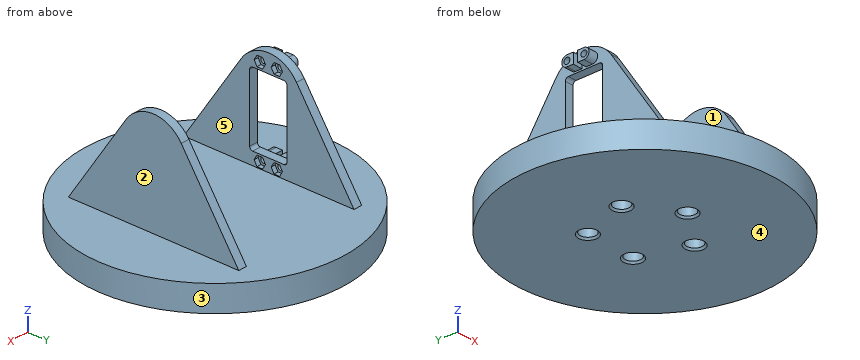
```python
from build123d import *

# Parameters (mm, degrees)
SKETCH1_R           = 75
BASE_PLATE_DEPTH    = 15
SKETCH2_R           = 4.5
DRIVE_HOLES_DEPTH   = 10
CHAMFER1_SIZE       = 1
BASE_START          = 40
BASE_FIN_DEPTH      = 5
BASE_START_2        = 70
BASE_FIN_2_DEPTH    = 5
CUT_EXTRUDE1_REACH  = 158.203
CUT_EXTRUDE2_REACH  = 158.203
SKETCH7_R           = 1.75
BOSS_EXTRUDE1_DEPTH = 5.6
CUT_EXTRUDE3_START  = -5.6
SKETCH9_R           = 1.75
CUT_EXTRUDE3_DEPTH  = 5.6
SKETCH10_W          = 4.6
SKETCH10_H          = 2.5
SKETCH10_W_2        = 6
CUT_EXTRUDE4_DEPTH  = 5.6
CUT_EXTRUDE5_DEPTH  = 2.6


with BuildPart() as part:
    # Sketch1 → Base Plate (new body)
    with BuildSketch(Plane.XY):
        Circle(SKETCH1_R)
    extrude(amount=BASE_PLATE_DEPTH)

    # Sketch2 → Drive Holes (cut)
    with BuildSketch(Plane(origin=(0, 0, 0), x_dir=(-1, 0, 0), z_dir=(0, 0, -1))):
        with Locations((0, -25)):
            Circle(SKETCH2_R)
        with Locations((-23.776412907, -7.725424859)):
            Circle(SKETCH2_R)
        with Locations((-14.694631307, 20.225424859)):
            Circle(SKETCH2_R)
        with Locations((14.694631307, 20.225424859)):
            Circle(SKETCH2_R)
        with Locations((23.776412907, -7.725424859)):
            Circle(SKETCH2_R)
    extrude(amount=-DRIVE_HOLES_DEPTH, mode=Mode.SUBTRACT)

    # Chamfer1
    chamfer1_edges = [part.edges().sort_by_distance(p)[0] for p in [
        (28.276412907, -7.725424859, 0),
        (19.194631307, 20.225424859, 0),
        (-10.194631307, 20.225424859, 0),
        (-19.276412907, -7.725424859, 0),
        (4.5, -25, 0),
    ]]
    chamfer(chamfer1_edges, length=CHAMFER1_SIZE)

    # Sketch4 → Base Fin (add)
    with BuildSketch(Plane(origin=(0, 0, 0), x_dir=(0, 0, -1), z_dir=(1, 0, 0)).offset(BASE_START)):
        with BuildLine():
            Line((-15, 50), (-65.791986374, 16.233382914))
            ThreePointArc((-65.791986374, 16.233382914), (-74.493324261, 0), (-65.791986374, -16.233382914))
            Line((-65.791986374, -16.233382914), (-15, -50))
            Line((-15, -50), (-15, 50))
        make_face()
    extrude(amount=-BASE_FIN_DEPTH)

    # Sketch5 → Base Fin 2 (add)
    with BuildSketch(Plane.ZY.offset(-35).offset(BASE_START_2)):
        with BuildLine():
            Line((15, 50), (15, -50))
            Line((15, -50), (65.791986374, -16.233382914))
            ThreePointArc((65.791986374, -16.233382914), (74.493324261, 0), (65.791986374, 16.233382914))
            Line((65.791986374, 16.233382914), (15, 50))
        make_face()
    extrude(amount=BASE_FIN_2_DEPTH)

    # Sketch6 → Cut-Extrude1 (cut, up to next)
    with BuildSketch(Plane.ZY.offset(40), mode=Mode.PRIVATE) as cut_extrude1_sk1:
        with BuildLine():
            Line((64, 8.875345998), (64, -9.524654002))
            ThreePointArc((64, -9.524654002), (63.487436867, -10.762090869), (62.25, -11.274654002))
            Line((62.25, -11.274654002), (24.05, -11.274654002))
            ThreePointArc((24.05, -11.274654002), (22.812563133, -10.762090869), (22.3, -9.524654002))
            Line((22.3, -9.524654002), (22.3, 8.875345998))
            ThreePointArc((22.3, 8.875345998), (22.812563133, 10.112782865), (24.05, 10.625345998))
            Line((24.05, 10.625345998), (62.25, 10.625345998))
            ThreePointArc((62.25, 10.625345998), (63.487436867, 10.112782865), (64, 8.875345998))
        make_face()
    cut_extrude1_tool1 = extrude(cut_extrude1_sk1.sketch, amount=-CUT_EXTRUDE1_REACH, mode=Mode.PRIVATE) & part.part
    add(cut_extrude1_tool1.solids().sort_by_distance((-40, -0.324654, 43.15))[0], mode=Mode.SUBTRACT)

    # Sketch7 → Cut-Extrude2 (cut, up to next)
    with BuildSketch(Plane.ZY.offset(40), mode=Mode.PRIVATE) as cut_extrude2_sk1:
        with Locations((18.35, 4.675345998)):
            Circle(SKETCH7_R)
    cut_extrude2_tool1 = extrude(cut_extrude2_sk1.sketch, amount=-CUT_EXTRUDE2_REACH, mode=Mode.PRIVATE) & part.part
    # Sketch7 → Cut-Extrude2 (cut, up to next)
    with BuildSketch(Plane.ZY.offset(40), mode=Mode.PRIVATE) as cut_extrude2_sk2:
        with Locations((18.35, -5.324654002)):
            Circle(SKETCH7_R)
    cut_extrude2_tool2 = extrude(cut_extrude2_sk2.sketch, amount=-CUT_EXTRUDE2_REACH, mode=Mode.PRIVATE) & part.part
    # Sketch7 → Cut-Extrude2 (cut, up to next)
    with BuildSketch(Plane.ZY.offset(40), mode=Mode.PRIVATE) as cut_extrude2_sk3:
        with Locations((67.95, -5.324654002)):
            Circle(SKETCH7_R)
    cut_extrude2_tool3 = extrude(cut_extrude2_sk3.sketch, amount=-CUT_EXTRUDE2_REACH, mode=Mode.PRIVATE) & part.part
    # Sketch7 → Cut-Extrude2 (cut, up to next)
    with BuildSketch(Plane.ZY.offset(40), mode=Mode.PRIVATE) as cut_extrude2_sk4:
        with Locations((67.95, 4.675345998)):
            Circle(SKETCH7_R)
    cut_extrude2_tool4 = extrude(cut_extrude2_sk4.sketch, amount=-CUT_EXTRUDE2_REACH, mode=Mode.PRIVATE) & part.part
    add(cut_extrude2_tool1.solids().sort_by_distance((-40, 4.675346, 18.35))[0], mode=Mode.SUBTRACT)
    add(cut_extrude2_tool2.solids().sort_by_distance((-40, -5.324654, 18.35))[0], mode=Mode.SUBTRACT)
    add(cut_extrude2_tool3.solids().sort_by_distance((-40, -5.324654, 67.95))[0], mode=Mode.SUBTRACT)
    add(cut_extrude2_tool4.solids().sort_by_distance((-40, 4.675346, 67.95))[0], mode=Mode.SUBTRACT)

    # Sketch8 → Boss-Extrude1 (add)
    with BuildSketch(Plane.ZY.offset(40)):
        with BuildLine():
            Line((70.95, 4.675345998), (70.95, -5.324654002))
            ThreePointArc((70.95, -5.324654002), (67.95, -8.324654002), (64.95, -5.324654002))
            Line((64.95, -5.324654002), (64.95, 4.675345998))
            ThreePointArc((64.95, 4.675345998), (67.95, 7.675345998), (70.95, 4.675345998))
        make_face()
        with BuildLine():
            Line((15, 7.675345998), (15, 0))
            Line((15, 0), (15, -8.324654002))
            Line((15, -8.324654002), (18.35, -8.324654002))
            ThreePointArc((18.35, -8.324654002), (20.471320344, -7.445974346), (21.35, -5.324654002))
            Line((21.35, -5.324654002), (21.35, 4.675345998))
            ThreePointArc((21.35, 4.675345998), (20.471320344, 6.796666341), (18.35, 7.675345998))
            Line((18.35, 7.675345998), (15, 7.675345998))
        make_face()
    extrude(amount=BOSS_EXTRUDE1_DEPTH)

    # Sketch9 → Cut-Extrude3 (cut)
    with BuildSketch(Plane(origin=(-40, 0, 0), x_dir=(0, 0, -1), z_dir=(1, 0, 0)).offset(CUT_EXTRUDE3_START)):
        with Locations(Location((-67.95, -5.324654002, 0), (0, 0, 180))):
            Circle(SKETCH9_R)
        with Locations(Location((-67.95, 4.675345998, 0), (0, 0, 180))):
            Circle(SKETCH9_R)
        with Locations(Location((-18.35, -5.324654002, 0), (0, 0, 180))):
            Circle(SKETCH9_R)
        with Locations(Location((-18.35, 4.675345998, 0), (0, 0, 180))):
            Circle(SKETCH9_R)
    extrude(amount=CUT_EXTRUDE3_DEPTH, mode=Mode.SUBTRACT)

    # Sketch10 → Cut-Extrude4 (cut)
    with BuildSketch(Plane.ZY.offset(45.6)):
        with Locations((19.05, -0.324654002)):
            Rectangle(SKETCH10_W, SKETCH10_H)
        with Locations((67.95, -0.324654002)):
            Rectangle(SKETCH10_W_2, SKETCH10_H)
    extrude(amount=-CUT_EXTRUDE4_DEPTH, mode=Mode.SUBTRACT)

    # Sketch11 → Cut-Extrude5 (cut)
    with BuildSketch(Plane(origin=(-35, 0, 0), x_dir=(0, 0, -1), z_dir=(1, 0, 0))):
        Polygon((-67.94416086, -2.00489509), (-70.822075983, -3.659717702), (-70.827915123, -6.979476615), (-67.95583914, -8.644412915), (-65.077924017, -6.989590302), (-65.072084877, -3.66983139), align=None)
        Polygon((-67.95, 7.995110046), (-70.825, 6.335228022), (-70.825, 3.015463974), (-67.95, 1.35558195), (-65.075, 3.015463974), (-65.075, 6.335228022), align=None)
        Polygon((-18.353543237, -2.004891845), (-21.226769981, -3.667841457), (-21.223226744, -6.987603614), (-18.346456763, -8.644416159), (-15.473230019, -6.981466547), (-15.476773256, -3.66170439), align=None)
        Polygon((-18.355430794, 7.995105604), (-21.22771155, 6.330522595), (-21.222280756, 3.010762989), (-18.344569206, 1.355586392), (-15.47228845, 3.020169401), (-15.477719244, 6.339929006), align=None)
    extrude(amount=-CUT_EXTRUDE5_DEPTH, mode=Mode.SUBTRACT)


solid = part.part
```
Geometry check sheet. Reference: the model listing, model coordinates, mm. Face numbers are marked on the shaded views. A direction names the side the tool comes from. Coordinates: 2 decimals unless noted, no trailing zeros. Order: outer loops, then holes, each group sorted by start corner. A loop starts at its lowest first (then second) coordinate and runs counter-clockwise, first axis right, second up. Notation, with made-up numbers: (83.5, 37) - (92.5, 37) arc R16 cw to (92.5, 53) - close; hole circle Ø7 at (61, -15.5). An arc over 180 degrees is marked (long way). Use one line per item in the form item = value.
1. Draft check along X on the marked faces 3, 4 and 5. Enter one of: pulls with the +X half, pulls with the -X half, needs draft (parallel to the pull), parting line crosses it, or undercut.
Here are the results:
face_3 = parting line crosses it
face_4 = needs draft
face_5 = undercut
2. Section check B-B (z = 6). Record the boundary of the cut face in (x, y).
Here are the results:
outline = circle Ø150 at (0, 0); hole circle Ø9 at (-23.78, -7.73); hole circle Ø9 at (-14.69, 20.23); hole circle Ø9 at (0, -25); hole circle Ø9 at (14.69, 20.23); hole circle Ø9 at (23.78, -7.73)
3. Section check D-D (x = -32.5). Record the boundary of the cut face in (y, z), then the cut area to 3 significant figures.
Here are the results:
outline = (-67.59, 0) - (67.59, 0) - (67.59, 15) - (-67.59, 15) - close
area = 2,030 mm²
4. Scan lines: line 1 (X direction, y = -44, z = 18); line 2 (Y direction, x = -39.4, z = 18.35); line 3 (Y direction, x = -37, z = 65.5). Record each from-to range of solid material in increasing order.
Here are the results:
line_1 = -40 to -35, 35 to 40
line_2 = -47.77 to -7.07, -3.57 to 2.93, 6.43 to 47.77
line_3 = -16.43 to -7.23, -3.42 to 2.77, 6.58 to 16.43
5. Access from +Z, -Z, +X, -X, +Y, -Y to the whole of each face (thin tool, end or side, straight path). Record for the marked faces 1 and 2.
Here are the results:
face_1 = +Z, +Y, -Y
face_2 = +Z, +X, +Y, -Y
6. Section check C-C (y = -25). Record the boundary of the cut face in (x, z), then the cut area to 3 significant figures.
Here are the results:
outline = (-70.71, 0) - (-5.5, 0) - (-4.5, 1) - (-4.5, 10) - (4.5, 10) - (4.5, 1) - (5.5, 0) - (70.71, 0) - (70.71, 15) - (40, 15) - (40, 52.61) - (35, 52.61) - (35, 15) - (-35, 15) - (-35, 52.61) - (-40, 52.61) - (-40, 15) - (-70.71, 15) - close
area = 2,410 mm²
7. Gauge pin test, flat ends, axial feed: pin 1 (6 mm diameter, centred on x = -41.5, z = 69.5, fed in from -Y); pin 2 (3 mm diameter, centred on x = -43.5, y = 3.5, fed in from +Z); pin 3 (3 mm diameter, centred on x = -0.5, y = -46, fed in from +Z). Record the tip position at first contact, or that the pin passes through.
Here are the results:
pin_1 = -15.44
pin_2 = 70.95
pin_3 = 15
8. Section check A-A (z = 45). Record the boundary of the cut face in (x, y), then the cut area to 3 significant figures.
Here are the results:
outline = (-40, -30.06) - (-35, -30.06) - (-35, -11.27) - (-40, -11.27) - close; (-40, 10.63) - (-35, 10.63) - (-35, 30.06) - (-40, 30.06) - close; (35, -30.06) - (40, -30.06) - (40, 30.06) - (35, 30.06) - close
area = 492 mm²
